Input: part model. Units: mm. Frame: model coordinates. Face numbers are marked on the shaded views. Coordinates: 2 decimals unless noted, no trailing zeros. Write each loop counter-clockwise with the first axis right and the second up, starting at its lowest first coordinate (ties: lowest second). Pieces come first, ordered by that corner, then holes. Notation, with made-up numbers: M -37,-19 L 2,-19 A23 ccw 2,19 Z; hole C -22,11.5 d3. An arc over 180 degrees is marked long. Use one line per item in the form item = value.
from build123d import *

# Parameters (mm, degrees)
CROQUIS1_R              = 4.75
SALIENTE_EXTRUIR1_DEPTH = 4


with BuildPart() as part:
    # Croquis1 → Saliente-Extruir1 (new body)
    # profile 1 of 2: a face of its own
    with BuildSketch(Plane.XY):
        Circle(CROQUIS1_R)
        with BuildLine():
            ThreePointArc((-2.1875, 1.210307296), (-1.767766953, 1.767766953), (-1.210307296, 2.1875))
            ThreePointArc((-1.210307296, 2.1875), (-0.157505366, 3.74003712), (1.25, 2.5))
            ThreePointArc((1.25, 2.5), (1.24003712, 2.342494634), (1.210307296, 2.1875))
            ThreePointArc((1.210307296, 2.1875), (1.767766953, 1.767766953), (2.1875, 1.210307296))
            ThreePointArc((2.1875, 1.210307296), (3.265465545, 0.988211769), (3.75, 0))
            ThreePointArc((3.75, 0), (3.265465545, -0.988211769), (2.1875, -1.210307296))
            ThreePointArc((2.1875, -1.210307296), (1.767766953, -1.767766953), (1.210307296, -2.1875))
            ThreePointArc((1.210307296, -2.1875), (1.24003712, -2.342494634), (1.25, -2.5))
            ThreePointArc((1.25, -2.5), (-0.157505366, -3.74003712), (-1.210307296, -2.1875))
            ThreePointArc((-1.210307296, -2.1875), (-1.767766953, -1.767766953), (-2.1875, -1.210307296))
            ThreePointArc((-2.1875, -1.210307296), (-3.75, 0), (-2.1875, 1.210307296))
        make_face(mode=Mode.SUBTRACT)
    # profile 2 of 2: a face of its own
    with BuildSketch(Plane.XY):
        with BuildLine():
            ThreePointArc((1.210307296, 2.1875), (0, 1.25), (-1.210307296, 2.1875))
            ThreePointArc((-1.210307296, 2.1875), (-1.767766953, 1.767766953), (-2.1875, 1.210307296))
            ThreePointArc((-2.1875, 1.210307296), (-1.511788231, 0.765465545), (-1.25, 0))
            ThreePointArc((-1.25, 0), (-1.511788231, -0.765465545), (-2.1875, -1.210307296))
            ThreePointArc((-2.1875, -1.210307296), (-1.767766953, -1.767766953), (-1.210307296, -2.1875))
            ThreePointArc((-1.210307296, -2.1875), (0, -1.25), (1.210307296, -2.1875))
            ThreePointArc((1.210307296, -2.1875), (1.767766953, -1.767766953), (2.1875, -1.210307296))
            ThreePointArc((2.1875, -1.210307296), (1.25, 0), (2.1875, 1.210307296))
            ThreePointArc((2.1875, 1.210307296), (1.767766953, 1.767766953), (1.210307296, 2.1875))
        make_face()
    extrude(amount=SALIENTE_EXTRUIR1_DEPTH)


solid = part.part
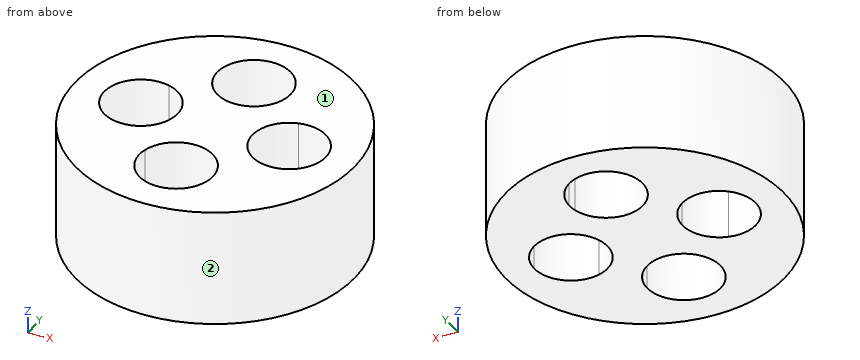
(1) Section query B-B on z = 0.8. Return the cut outline in (x, y), plus the area to 3 significant figures.
Computed:
outline = C 0,0 d9.5; hole C -2.5,0 d2.5; hole C 0,-2.5 d2.5; hole C 0,2.5 d2.5; hole C 2.5,0 d2.5
area = 51.2 mm^2
(2) Pull-direction query (Y, two-part tool) for the marked faces 1 and 2; classes: pulls with the +Y half, pulls with the -Y half, needs draft (parallel to the pull), parting line crosses it, or undercut.
Computed:
face_1 = needs draft
face_2 = parting line crosses it
(3) Section query A-A on x = 0. Return the cut outline in (y, z), plus the area to 3 significant figures.
Computed:
outline = M -4.75,0 L -3.75,0 L -3.75,4 L -4.75,4 Z; M -1.25,0 L 1.25,0 L 1.25,4 L -1.25,4 Z; M 3.75,0 L 4.75,0 L 4.75,4 L 3.75,4 Z
area = 18.0 mm^2
(4) Line query: probe 1 along X at (y, z) = (-1, 2.5); probe 2 along X at (y, z) = (-2.5, 0.4); probe 3 along Y at (x, z) = (-2, 3.55). Output: solid intervals per line, ascending.
Computed:
probe_1 = -4.64 to -3.25, -1.75 to 1.75, 3.25 to 4.64
probe_2 = -4.04 to -1.25, 1.25 to 4.04
probe_3 = -4.31 to -1.15, 1.15 to 4.31
(5) Section query C-C on y = 3.25. Return the cut outline in (x, z), plus the area to 3 significant figures.
Computed:
outline = M -3.46,0 L -1,0 L -1,4 L -3.46,4 Z; M 1,0 L 3.46,0 L 3.46,4 L 1,4 Z
area = 19.7 mm^2
(6) First-contact query: pin 1 Ø3 at (x, y) = (0, 2.5) entering from -Z; pin 2 Ø1 at (x, z) = (2.5, 3.5) entering from -Y. Flat tips, straight axial feed; report the tip coordinate or a pass-through.
Computed:
pin_1 = 0
pin_2 = -4.31
(7) Section query D-D on x = 1.75. Return the cut outline in (y, z).
Computed:
outline = M -4.42,0 L -1,0 L -1,4 L -4.42,4 Z; M 1,0 L 4.42,0 L 4.42,4 L 1,4 Z
